Build history of the part. All positions in model axes, mm. Round coordinates to 2 decimals unless told otherwise and drop trailing zeros. Write each loop counter-clockwise with the first axis right and the second up, starting at its lowest first coordinate (ties: lowest second). Pieces come first, ordered by that corner, then holes.
Item 1: Wall check: probe 1 along Y at (x, z) = (-63.5, 1.45); probe 2 along Y at (x, z) = (-93, 1.7); probe 3 along X at (y, z) = (41, 2.75). Give the ranges that are in metal, low to high.
Item 2: Band-saw the part on C-C, the plane z = 1.1. Count the separate pieces of the cut face and the enclosed holes in it, then the cut area to 3 significant figures.
Item 3: Band-saw the part on A-A, the plane y = 76.2. Write the cut outline in (x, z) (1 decimal), then the cut area to 3 significant figures.
Item 4: Band-saw the part on B-B, the plane x = -64.5. Write the cut outline in (y, z) (3 decimals).
Item 5: Band-saw the part on D-D, the plane x = -94. Write the cut outline in (y, z) (3 decimals), then the cut area to 3 significant figures.
Item 6: Drop flat-ended pins along their axis: pin 1 Ø1 at (x, z) = (-39, 0.5) entering from +Y; pin 2 Ø1 at (y, z) = (85.5, 2) entering from -X; pin 3 Ø1 at (x, z) = (6.5, 2) entering from -Y; pin 4 Ø5 at (x, y) = (-55.11, 223.39) entering from -Z. Give the stop position or say it passes through.
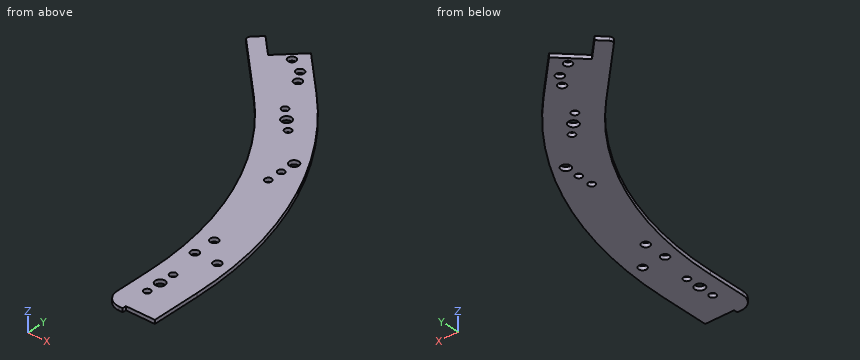
Autodesk Inventor part; units mm, degrees
ref_plane "YZ Plane" through (0, 0, 0) normal (1, 0, 0) x (0, 1, 0)
ref_plane "XZ Plane" through (0, 0, 0) normal (0, 1, 0) x (-1, 0, 0)
ref_plane "XY Plane" through (0, 0, 0) normal (0, 0, 1) x (1, 0, 0)
sketch "Sketch1" plane through (0, 0, 0) normal (0, 0, 1) x (1, 0, 0)
  arc A0 (-15.749, 9.525) -> (-3.049, -3.175) centre (-3.049, 9.525) ccw
  line L0 (-3.049, -3.175) -> (0, -3.175)
  line L1 (0, -3.175) -> (0, 0)
  line L2 (0, 0) -> (24.5753, 0)
  line L3 (24.5753, 0) -> (24.5753, 41.4619)
  arc A1 (24.5753, 41.4619) -> (-69.0697, 267.5412) centre (-295.149, 41.4619) ccw
  line L4 (-69.0697, 267.5412) -> (-102.8779, 301.3493)
  line L5 (-102.8779, 301.3493) -> (-122.4112, 281.816)
  line L6 (-122.4112, 281.816) -> (-138.1267, 297.5314)
  line L7 (-138.1267, 297.5314) -> (-144.8619, 290.7962)
  arc A2 (-144.8619, 290.7962) -> (-144.8619, 286.3061) centre (-142.6168, 288.5511) ccw
  line L8 (-144.8619, 286.3061) -> (-97.5834, 239.0276)
  arc A3 (-15.749, 41.4619) -> (-97.5834, 239.0276) centre (-295.149, 41.4619) ccw
  line L9 (-15.749, 41.4619) -> (-15.749, 9.525)
  circle A4 centre (-1.0086, 22.225) radius 2.8448
  circle A5 centre (-1.0086, 47.625) radius 2.8448
  circle A6 centre (-26.9212, 171.2375) radius 2.85
  circle A7 centre (-26.9212, 183.9375) radius 2.85
  circle A8 centre (-26.9212, 196.6375) radius 4
  circle A9 centre (-73.0746, 241.3501) radius 2.85
  circle A10 centre (-55.1141, 223.3895) radius 2.85
  circle A11 centre (-7.1747, 76.2) radius 3.3782
  circle A12 centre (11.8753, 76.2) radius 3.3782
  circle A13 centre (-7.1747, 95.25) radius 3.3782
  circle A14 centre (-107.368, 287.8789) radius 3.3782
  circle A15 centre (-94.108, 280.5097) radius 3.3782
  circle A16 centre (-87.758, 270.9847) radius 3.3782
  circle A17 centre (-1.0086, 34.925) radius 4.15
  circle A18 centre (-64.0943, 232.3698) radius 4.15
  line L10 (-97.5834, 239.0276) -> (-69.0697, 267.5412) construction
  line L11 (-15.749, 41.4619) -> (24.5753, 41.4619) construction
  line L12 (-1.0086, 47.625) -> (-1.0086, 22.225) construction
  line L13 (-7.1747, 76.2) -> (11.8753, 76.2) construction
  line L14 (-7.1747, 76.2) -> (-7.1747, 95.25) construction
  line L15 (-26.9212, 196.6375) -> (-26.9212, 171.2375) construction
  line L16 (-73.0746, 241.3501) -> (-55.1141, 223.3895) construction
  dimension "d0" = 279.4
  dimension "d1" = 319.7243
  dimension "d2" = 6.7564
  dimension "d3" = 6.7564
  dimension "d4" = 6.7564
  dimension "d5" = 5.7
  dimension "d6" = 8.3
  dimension "d7" = 5.7
  dimension "d8" = 8
  dimension "d9" = 5.7
  dimension "d10" = 5.7
  dimension "d11" = 3.175
  dimension "d12" = 12.7
  dimension "d13" = 22.225
  dimension "d14" = 27.6243
  dimension "d15" = 47.8119
  dimension "d16" = 70.0369
  dimension "d17" = 66.8619
  dimension "d18" = 45
  dimension "d19" = 6.7564
  dimension "d20" = 6.7564
  dimension "d21" = 6.7564
  dimension "d22" = 5.6896
  dimension "d23" = 8.3
  dimension "d24" = 5.6896
  dimension "d25" = 12.7
  dimension "d26" = 3.049
  dimension "d27" = 24.5753
  dimension "d28" = 3.175
  dimension "d29" = 41.4619
  dimension "d30" = 31.9369
  dimension "d32" = 14.7404
  dimension "d33" = 22.225
  dimension "d34" = 34.7381
  dimension "d35" = 19.05
  dimension "d36" = 19.05
  dimension "d37" = 8.5743
  dimension "d38" = 11.1722
  dimension "d39" = 171.2375
  dimension "d40" = 18.9726
  dimension "d41" = 63.5
  dimension "d42" = 6.35
  dimension "d43" = 12.7
  dimension "d44" = 8.5346
  dimension "d46" = 20.9371
  dimension "d48" = 25.4
  dimension "d49" = 25.4
  dimension "d50" = 25.4
  dimension "d53" = 6.35
  dimension "d54" = 9.525
extrude "Extrusion1" add sketch "Sketch1" along normal blind 3.175
properties part number "V5 Shooter Conveyor Plate P1 (45 Deg)" material "Aluminum-6061"
Results:
1. probe 1: y = 197.68 to 228.26, 236.48 to 261.83
1. probe 2: y = 234.34 to 277.32, 283.7 to 291.47
1. probe 3: x = -15.75 to 24.58
2. separate pieces: 1
2. enclosed holes: 15
2. area: 12,900 mm2
3. outline: (-17.9, 0) - (-10.6, 0) - (-10.6, 3.2) - (-17.9, 3.2) - close; (-3.8, 0) - (8.5, 0) - (8.5, 3.2) - (-3.8, 3.2) - close; (15.3, 0) - (22.7, 0) - (22.7, 3.2) - (15.3, 3.2) - close
3. area: 86.0 mm2
4. outline: (199.15, 0) - (228.24, 0) - (228.24, 3.175) - (199.15, 3.175) - close; (236.5, 0) - (262.877, 0) - (262.877, 3.175) - (236.5, 3.175) - close
5. outline: (235.378, 0) - (277.133, 0) - (277.133, 3.175) - (235.378, 3.175) - close; (283.886, 0) - (292.471, 0) - (292.471, 3.175) - (283.886, 3.175) - close
5. area: 160 mm2
6. pin 1: stops at y = 233.47
6. pin 2: stops at x = -19.32
6. pin 3: stops at y = 0
6. pin 4: passes through
